Read the model definition and answer for the solid it produces. Units are mm, in the model's axes. Face numbers are marked on the shaded views. A direction names the side the tool comes from. Coordinates: 2 decimals unless noted, no trailing zeros. Loops run counter-clockwise (first coordinate to the right, second up) from the corner with the lowest first, then second, coordinate; pieces in that order, holes last. Notation, with made-up numbers: (7, -14.5) - (33, -14.5) arc R24 ccw to (33, 11.5) - close; hole circle Ø9 at (52.25, 74.5). An arc over 180 degrees is marked (long way). Use CSV: the item, a comma, the result in double quotes.
```python
from build123d import *

# Parameters (mm, degrees)
SKETCH1_R           = 7.5
SKETCH1_R_2         = 1.75
BOSS_EXTRUDE1_DEPTH = 20
SKETCH2_W           = 3
SKETCH2_H           = 3
CUT_EXTRUDE1_DEPTH  = 8
CUT_EXTRUDE2_DEPTH  = 8


with BuildPart() as part:
    # Sketch1 → Boss-Extrude1 (new body)
    with BuildSketch(Plane.XY):
        Circle(SKETCH1_R)
        Circle(SKETCH1_R_2, mode=Mode.SUBTRACT)
    extrude(amount=BOSS_EXTRUDE1_DEPTH)

    # Sketch2 → Cut-Extrude1 (cut)
    with BuildSketch(Plane.XY.offset(20)):
        with Locations((0, 4.5)):
            Rectangle(SKETCH2_W, SKETCH2_H)
    extrude(amount=-CUT_EXTRUDE1_DEPTH, mode=Mode.SUBTRACT)

    # Sketch3 → Cut-Extrude2 (cut)
    with BuildSketch(Plane(origin=(0, 0, 0), x_dir=(-1, 0, 0), z_dir=(0, 0, -1))):
        Polygon((-0.499533791, 3.31669504), (0.427517192, 6.169864589), (3.280686741, 5.242813606), (2.353635758, 2.389644057), align=None)
    extrude(amount=-CUT_EXTRUDE2_DEPTH, mode=Mode.SUBTRACT)


solid = part.part
```
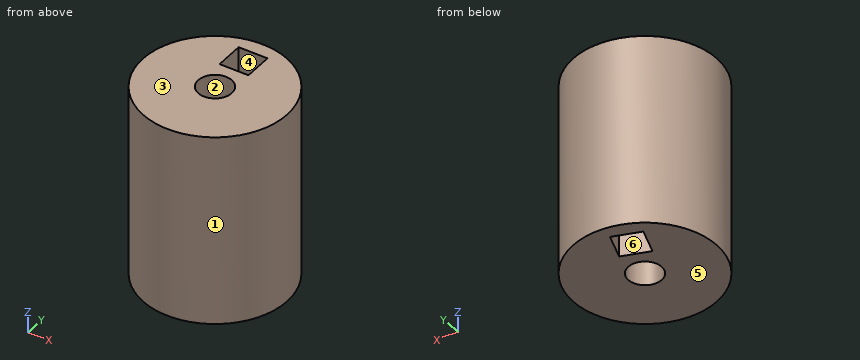
Q1. A tool of negligible diameter and unlimited length cuts with its end or side. For the marked faces 4, 5 and 6, from which of +Z, -Z, +X, -X, +Y, -Y can it reach the whole face along a straight path? Write none if from no direction.
Reported:
face 4,"+Z"
face 5,"-Z, +X, -X, +Y, -Y"
face 6,"-Z"
Q2. The part is cut by section C-C on x = 0. Determine the outline of the cut face in (y, z), and give its area (3 significant figures).
Reported:
outline,"(-7.5, 0) - (-1.75, 0) - (-1.75, 20) - (-7.5, 20) - close; (1.75, 0) - (3.15, 0) - (3.15, 8) - (4.85, 8) - (4.85, 0) - (7.5, 0) - (7.5, 20) - (6, 20) - (6, 12) - (3, 12) - (3, 20) - (1.75, 20) - close"
area,"192 mm²"
Q3. The part is cut by section A-A on z = 17.75. Determine the outline of the cut face in (x, y), and give its area (3 significant figures).
Reported:
outline,"circle Ø15 at (0, 0); hole circle Ø3.5 at (0, 0); hole (-1.5, 3) - (1.5, 3) - (1.5, 6) - (-1.5, 6) - close"
area,"158 mm²"
Q4. Find the intervals of material crossed by probe 1 along Y at (x, z) = (0, 16.25); probe 2 along Y at (x, z) = (0, 11.25); probe 3 along X at (y, z) = (-0.5, 19), in increasing order. Write a range as [from, to].
Reported:
probe 1,"y = [-7.5, -1.75], [1.75, 3], [6, 7.5]"
probe 2,"y = [-7.5, -1.75], [1.75, 7.5]"
probe 3,"x = [-7.48, -1.68], [1.68, 7.48]"
Q5. The part is cut by section B-B on y = 0. Determine the outline of the cut face in (x, z).
Reported:
outline,"(-7.5, 0) - (-1.75, 0) - (-1.75, 20) - (-7.5, 20) - close; (1.75, 0) - (7.5, 0) - (7.5, 20) - (1.75, 20) - close"
Q6. Given P1, Ø1, axis at x = -6, z = 7.5, coming from the -Y side; P2, Ø5, axis at x = 0.5, z = 3, coming from the +Y side; P3, Ø2.5, axis at y = 5, z = 15, coming from the +X side; P4, Ø3.5, axis at y = 4, z = 15, coming from the -X side, each flat-ended and moving along its own axis, determine where each tip first touches the part or whether it passes through.
Reported:
P1,"stops at y = -5.1"
P2,"stops at y = 7.5"
P3,"stops at x = 6.5"
P4,"stops at x = -7.15"
Q7. For a pull along X with two mould halves and no side action, classify the marked faces 1, 2 and 3 as +X half, -X half, draft (parallel to the pull), parting line (faces both ways), or undercut.
Reported:
face 1,"parting line"
face 2,"undercut"
face 3,"draft"
Q8. The part is cut by section D-D on z = 9.5. Determine the outline of the cut face in (x, y), and give its area (3 significant figures).
Reported:
outline,"circle Ø15 at (0, 0); hole circle Ø3.5 at (0, 0)"
area,"167 mm²"
